from build123d import *

# Parameters (mm, degrees)
BOSS_EXTRUDE1_DEPTH  = 2
SKETCH2_R            = 5
BOSS_EXTRUDE2_DEPTH  = 4
M4_CLEARANCE_HOLE1_D = 4.5


with BuildPart() as part:
    # Sketch1 → Boss-Extrude1 (new, symmetric)
    with BuildSketch(Plane.XY):
        with BuildLine():
            Line((0, 5), (69.15, 5))
            ThreePointArc((69.15, 5), (74.15, 0), (69.15, -5))
            Line((69.15, -5), (0, -5))
            ThreePointArc((0, -5), (-5, 0), (0, 5))
        make_face()
    extrude(amount=BOSS_EXTRUDE1_DEPTH, both=True)

    # Sketch2 → Boss-Extrude2 (add, symmetric)
    with BuildSketch(Plane.XY.offset(2)):
        with Locations(Location((0, 0, 0), (0, 0, 270))):
            Circle(SKETCH2_R)
    extrude(amount=BOSS_EXTRUDE2_DEPTH, both=True)

    # M4 Clearance Hole1 (through all)
    with Locations(Plane(origin=(0, 0, -2), x_dir=(-1, 0, 0), z_dir=(0, 0, -1))):
        with Locations((-69.15, 0)):
            Hole(M4_CLEARANCE_HOLE1_D / 2)


solid = part.part
Read the model definition and answer for the solid it produces. Units are mm, in the model's axes. Round coordinates to 2 decimals unless told otherwise and drop trailing zeros. Order: outer loops, then holes, each group sorted by start corner. A loop starts at its lowest first (then second) coordinate and runs counter-clockwise, first axis right, second up.
1) The mould has two halves that part along Y. Classify faces 1 (the face through (66.902, 0.099, 0.028)), 2 (the face through (-4.957, 0.651, 2.945)), 3 (the face through (35, 0, -2)), 4 (the face through (34, 5, 0)): released by +Y, released by -Y, zero draft, split by the parting line, or undercut.
2) The part is cut by section C-C on x = 9. Write down the section's boundary in (y, z), plus the area to 3 significant figures.
3) The part is cut by section A-A on y = 0. Write down the section's boundary in (x, z).
4) The part is cut by section B-B on z = 0.75. Write down the section's boundary in (x, y), plus the area to 3 significant figures.
5) Flat-ended cylindrical pins translate along their axes: pin 1 (1.5 mm diameter, centred on y = 1, z = 3, fed in from +X); pin 2 (1 mm diameter, centred on y = 3.5, z = 2, fed in from -X); pin 3 (1.5 mm diameter, centred on y = 2.5, z = 4.5, fed in from +X). Find the tip coordinate at first contact, or state that the pin passes through.
6) Straight lines are drawn through the part: L1, parallel to Y at x = 69.15, z = 0.45; L2, parallel to Z at x = 9.5, y = 1.5; L3, parallel to X at y = 1.75, z = -1.25. For each, find the intervals that lie inside material, in ascending order.
7) The part is cut by section D-D on z = 5.25. Write down the section's boundary in (x, y), plus the area to 3 significant figures.
Resolved:
1. face 1: undercut
1. face 2: split by the parting line
1. face 3: zero draft
1. face 4: released by +Y
2. outline: (-5, -2) - (5, -2) - (5, 2) - (-5, 2) - close
2. area: 40.0 mm2
3. outline: (-5, -2) - (66.9, -2) - (66.9, 2) - (5, 2) - (5, 6) - (-5, 6) - close; (71.4, -2) - (74.15, -2) - (74.15, 2) - (71.4, 2) - close
4. outline: (0, -5) - (69.15, -5) arc R5 ccw to (69.15, 5) - (0, 5) arc R5 ccw to start; hole circle Ø4.5 at (69.15, 0)
4. area: 754 mm2
5. pin 1: stops at x = 4.99
5. pin 2: stops at x = -4
5. pin 3: stops at x = 4.68
6. L1: y = -5 to -2.25, 2.25 to 5
6. L2: z = -2 to 2
6. L3: x = -4.68 to 67.74, 70.56 to 73.83
7. outline: circle Ø10 at (0, 0)
7. area: 78.5 mm2
